```python
from build123d import *

# Parameters (mm, degrees)
F1_DEPTH = 228.6
F2_R     = 25.4
F3_DEPTH = 228.601
F4_T     = -3.4163
F5_R     = 6.35
F6_R     = 3.175


with BuildPart() as f1:
    # F0 (on Front) → F1 (new body)
    with BuildSketch(Plane.XZ):
        with BuildLine():
            Line((101.6, 152.4), (-101.6, 152.4))
            ThreePointArc((-101.6, 152.4), (-119.5605122421, 144.9605122421), (-127, 127))
            Line((-127, 127), (-127, 0))
            Line((-127, 0), (127, 0))
            Line((127, 0), (127, 127))
            ThreePointArc((127, 127), (119.5605122421, 144.9605122421), (101.6, 152.4))
        make_face()
    extrude(amount=F1_DEPTH)

    # F2 (on face) → F3 (cut, through all)
    with BuildSketch(Plane.XZ.offset(228.6)):
        with Locations((-76.2, 76.2)):
            Circle(F2_R)
        with Locations((50.8, 76.2)):
            Circle(F2_R)
    extrude(amount=-F3_DEPTH, mode=Mode.SUBTRACT)

    # F4
    f4_openings = [f1.faces().sort_by_distance(p)[0] for p in [
        (127, -114.3, 63.5),
        (119.560512, -114.3, 144.960512),
        (0, -114.3, 152.4),
        (-127, -114.3, 63.5),
        (-119.560512, -114.3, 144.960512),
        (-101.6, -114.3, 76.2),
        (25.4, -114.3, 76.2),
    ]]
    offset(amount=F4_T, openings=f4_openings)

    # F5
    f5_edges = [f1.edges().sort_by_distance(p)[0] for p in [
        (0, 0, 0),
        (0, -228.6, 0),
    ]]
    fillet(f5_edges, radius=F5_R)

    # F6
    f6_edges = [f1.edges().sort_by_distance(p)[0] for p in [
        (0, -3.4163, 3.4163),
        (0, -225.1837, 3.4163),
    ]]
    fillet(f6_edges, radius=F6_R)


solid = f1.part
```
Geometry: final body of the model. Coordinates: model frame, mm. A direction names the side the tool comes from. Round coordinates to 2 decimals unless told otherwise and drop trailing zeros. Loops run counter-clockwise (first coordinate to the right, second up) from the corner with the lowest first, then second, coordinate; pieces in that order, holes last. Notation, with made-up numbers: (7.5, -25) -> (34.5, -25) arc R8 ccw to (34.5, -20) -> close; hole circle Ø3 at (1, -35.5). An arc over 180 degrees is marked (long way). Use one line per item in the form item = value.
Item 1: Cut plane D-D on y = -155.5. Output: boundary loops of the cut face in (x, z).
Evaluation:
outline = (-127, 0) -> (127, 0) -> (127, 3.42) -> (-127, 3.42) -> close
Item 2: Material intervals for probe 1 along X at (y, z) = (-2, 76); probe 2 along Y at (x, z) = (-65, 31); probe 3 along Z at (x, y) = (-101.5, -212), sorted ascending.
Evaluation:
probe_1 = -127 to -101.6, -50.8 to 25.4, 76.2 to 127
probe_2 = -228.6 to -225.18, -3.42 to 0
probe_3 = 0 to 3.42
Item 3: Contact query for flat-ended pins moving along their axis: pin 1 Ø5 at (x, y) = (7, -184.5) entering from +Z; pin 2 Ø10 at (x, z) = (-77.5, 121) entering from +Y. Output: stop coordinate, or through.
Evaluation:
pin_1 = 3.42
pin_2 = 0
Item 4: Access query for faces 1 (the flat face through (127, -114, 2)), 2 (the flat face through (-2, -3.416, 81)). Directions: +Z, -Z, +X, -X, +Y, -Y. A direction counts if a zero-diameter tool reaches every point of the face in a straight line with its end or side. Return the directions, or none.
Evaluation:
face_1 = +Z, -Z, +X, +Y, -Y
face_2 = +Z, +X, -X
Item 5: Draft query along X for faces 3 (the flat face through (-2, -225.184, 81)), 4 (the cylindrical face through (32.08, -1.73, 93.37)), 5 (the cylindrical face through (-79.507, -1.732, 101.384)), 6 (the cylindrical face through (119.76, -1.68, 144.76)). Return one class per face: released by +X, released by -X, zero draft, split by the parting line, or undercut.
Evaluation:
face_3 = zero draft
face_4 = undercut
face_5 = undercut
face_6 = released by +X
Item 6: Cut plane C-C on x = -22.5. Output: boundary loops of the cut face in (y, z) (3 decimals).
Evaluation:
outline = (-228.6, 6.35) arc R6.35 ccw to (-222.25, 0) -> (-6.35, 0) arc R6.35 ccw to (0, 6.35) -> (0, 152.4) -> (-3.416, 152.4) -> (-3.416, 6.591) arc R3.175 cw to (-6.591, 3.416) -> (-222.009, 3.416) arc R3.175 cw to (-225.184, 6.591) -> (-225.184, 152.4) -> (-228.6, 152.4) -> close
Item 7: Cut plane B-B on z = 76.2. Output: boundary loops of the cut face in (x, y), then the cut area to 3 significant figures.
Evaluation:
outline = (-127, -228.6) -> (-101.6, -228.6) -> (-101.6, -225.18) -> (-127, -225.18) -> close; (-127, -3.42) -> (-101.6, -3.42) -> (-101.6, 0) -> (-127, 0) -> close; (-50.8, -228.6) -> (25.4, -228.6) -> (25.4, -225.18) -> (-50.8, -225.18) -> close; (-50.8, -3.42) -> (25.4, -3.42) -> (25.4, 0) -> (-50.8, 0) -> close; (76.2, -228.6) -> (127, -228.6) -> (127, -225.18) -> (76.2, -225.18) -> close; (76.2, -3.42) -> (127, -3.42) -> (127, 0) -> (76.2, 0) -> close
area = 1,040 mm2
Item 8: Cut plane A-A on x = 50.8. Output: boundary loops of the cut face in (y, z) (3 decimals).
Evaluation:
outline = (-228.6, 6.35) arc R6.35 ccw to (-222.25, 0) -> (-6.35, 0) arc R6.35 ccw to (0, 6.35) -> (0, 50.8) -> (-3.416, 50.8) -> (-3.416, 6.591) arc R3.175 cw to (-6.591, 3.416) -> (-222.009, 3.416) arc R3.175 cw to (-225.184, 6.591) -> (-225.184, 50.8) -> (-228.6, 50.8) -> close; (-228.6, 101.6) -> (-225.184, 101.6) -> (-225.184, 152.4) -> (-228.6, 152.4) -> close; (-3.416, 101.6) -> (0, 101.6) -> (0, 152.4) -> (-3.416, 152.4) -> close
